from build123d import *


with BuildPart() as part:
    # Esboço1 → Revolução1 (revolve)
    with BuildSketch(Plane.XY, mode=Mode.PRIVATE) as revolu_o1_sk:
        Polygon((0, 75), (25, 75), (25, 50), (37.5, 50), (50, 0), (75, -25), (75, -50), (90, -50), (90, -75), (0, -75), align=None)
    revolve(revolu_o1_sk.sketch.rotate(Axis((0, 54.909632035, 0), (0, -1, 0)), 90), axis=Axis((0, 54.909632035, 0), (0, -1, 0)))  # turned: the seam where the file's is


solid = part.part
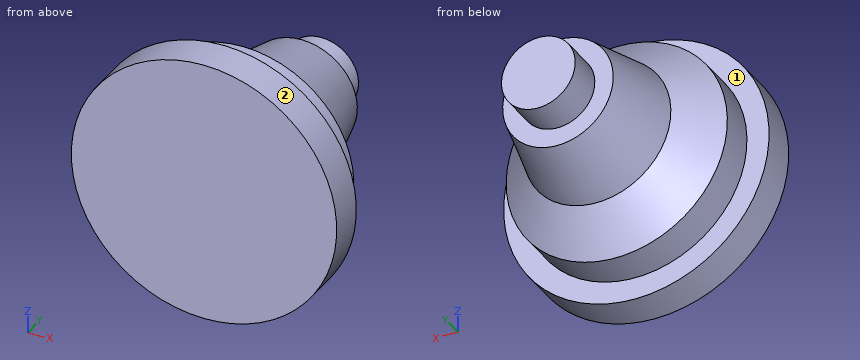
The listing builds one solid part. Answer for the finished solid, in the listing's coordinates (mm). Face numbers are marked on the shaded views. A direction names the side the tool comes from. Give positions to 0.01 mm unless a question says otherwise; leave off trailing zeros. Loops run counter-clockwise (first coordinate to the right, second up) from the corner with the lowest first, then second, coordinate; pieces in that order, holes last.
Item 1: A cutting plane is placed at A-A (x = 0). Give the vertices of the cut face in (y, z), then the cut area to 3 significant figures.
Derived:
outline: (-75, -90) - (-50, -90) - (-50, -75) - (-25, -75) - (0, -50) - (50, -37.5) - (50, -25) - (75, -25) - (75, 25) - (50, 25) - (50, 37.5) - (0, 50) - (-25, 75) - (-50, 75) - (-50, 90) - (-75, 90) - close
area: 17,000 mm2
Item 2: Each of these flat-tipped pins is pushed along its axis until it touches: pin 1 Ø2 at (x, y) = (-5.5, 29.5) entering from -Z; pin 2 Ø4 at (x, y) = (-19, 38.5) entering from -Z; pin 3 Ø10 at (x, y) = (-1, -12) entering from +Z. Where does it stop, or does it pass through?
Derived:
pin 1: stops at z = -42.55
pin 2: stops at z = -36.77
pin 3: stops at z = 66.99
Item 3: A cutting plane is placed at C-C (y = -61). Give the vertices of the cut face in (x, z).
Derived:
outline: circle Ø180 at (0, 0)
Item 4: A tool of negligible diameter and unlimited length cuts with its end or side. For the marked faces 1 and 2, from which of +Z, -Z, +X, -X, +Y, -Y can it reach the whole face along a straight path? Write none if from no direction.
Derived:
face 1: +Y
face 2: +Y, -Y
Item 5: Find the intervals of material crossed by line 1 along Y through (x, z) = (55, -60); line 2 along X through (y, z) = (-33, 44); line 3 along Z through (x, y) = (28, -2), in increasing order.
Derived:
line 1: y = -75 to -50
line 2: x = -60.74 to 60.74
line 3: z = -43.82 to 43.82
Item 6: A cutting plane is placed at D-D (x = 77.5). Give the vertices of the cut face in (y, z).
Derived:
outline: (-75, -45.76) - (-50, -45.76) - (-50, 45.76) - (-75, 45.76) - close
Item 7: A cutting plane is placed at B-B (z = 0). Give the vertices of the cut face in (x, y), then the cut area to 3 significant figures.
Derived:
outline: (-90, -75) - (90, -75) - (90, -50) - (75, -50) - (75, -25) - (50, 0) - (37.5, 50) - (25, 50) - (25, 75) - (-25, 75) - (-25, 50) - (-37.5, 50) - (-50, 0) - (-75, -25) - (-75, -50) - (-90, -50) - close
area: 17,000 mm2
